from build123d import *

# Parameters (mm, degrees)
SKETCH1_W            = 80
SKETCH1_H            = 193.756044748
BOSS_EXTRUDE1_DEPTH  = 4
M8_CLEARANCE_HOLE1_D = 8.4
M5_CLEARANCE_HOLE1_D = 5.3


with BuildPart() as part:
    # Sketch1 → Boss-Extrude1 (new body)
    with BuildSketch(Plane.XY):
        with Locations((1780.42117355, -1810.70620503)):
            Rectangle(SKETCH1_W, SKETCH1_H)
    extrude(amount=BOSS_EXTRUDE1_DEPTH)

    # M8 Clearance Hole1 (through all)
    with Locations(Plane.XY.offset(4)):
        with Locations((1757.421173548, -1767.419409116), (1803.421173548, -1767.419409116), (1803.421173548, -1785.419409116), (1757.421173548, -1785.419409116), (1800.42117355, -1841.919409116), (1760.42117355, -1841.919409116), (1800.42117355, -1881.919409116), (1760.42117355, -1881.919409116)):
            Hole(M8_CLEARANCE_HOLE1_D / 2)

    # M5 Clearance Hole1 (through all)
    with Locations(Plane.XY.offset(4)):
        with Locations((1813.754187213, -1767.419409116), (1747.088159883, -1767.419409116), (1780.421173548, -1734.086395451), (1780.421173548, -1800.752422781)):
            Hole(M5_CLEARANCE_HOLE1_D / 2)


solid = part.part
The listing builds one solid part. Answer for the finished solid, in the listing's coordinates (mm). Coordinates: 2 decimals unless noted, no trailing zeros. Order: outer loops, then holes, each group sorted by start corner. A loop starts at its lowest first (then second) coordinate and runs counter-clockwise, first axis right, second up.
Q1. A cutting plane is placed at A-A, the plane x = 1814.5. Write down the section's boundary in (y, z), and give its area (3 significant figures).
Q2. A cutting plane is placed at B-B, the plane z = 0.7. State how many separate pieces and enclosed holes the cut face has, and give its area (3 significant figures).
Q3. Consider line 1 (Y direction, x = 1781.5, z = 2.15); line 2 (Y direction, x = 1763, z = 1.5); line 3 (Y direction, x = 1759.5, z = 1.9). Determine where each line is inside the solid, lowest interval first.
Q4. For a pull along Y with two mould halves and no side action, classify faces 1 (the face through (1780, -1809, 4)), 2 (the face through (1780, -1713.828, 2)), 3 (the face through (1763.75, -1844.48, 1.97)), 4 (the face through (1780, -1907.584, 2)) as pulls with the +Y half, pulls with the -Y half, needs draft (parallel to the pull), parting line crosses it, or undercut.
Answers follow:
1. outline: (-1907.58, 0) - (-1769.96, 0) - (-1769.96, 4) - (-1907.58, 4) - close; (-1764.88, 0) - (-1713.83, 0) - (-1713.83, 4) - (-1764.88, 4) - close
1. area: 755 mm2
2. separate pieces: 1
2. enclosed holes: 12
2. area: 15,000 mm2
3. line 1: y = -1907.58 to -1803.17, -1798.33 to -1736.51, -1731.67 to -1713.83
3. line 2: y = -1907.58 to -1885.23, -1878.6 to -1845.23, -1838.6 to -1713.83
3. line 3: y = -1907.58 to -1886.02, -1877.82 to -1846.02, -1837.82 to -1789.07, -1781.77 to -1771.07, -1763.77 to -1713.83
4. face 1: needs draft
4. face 2: pulls with the +Y half
4. face 3: undercut
4. face 4: pulls with the -Y half
